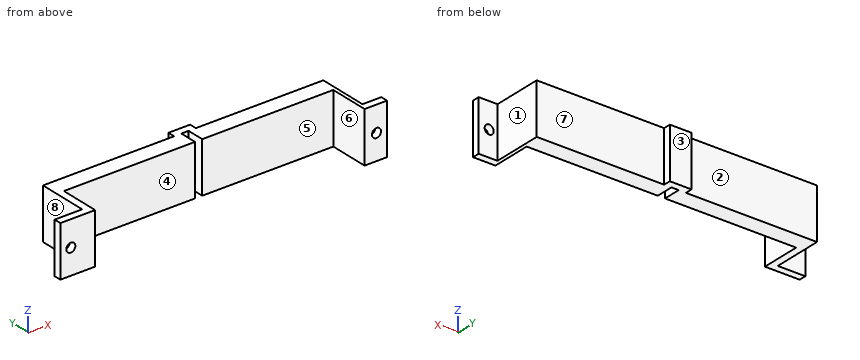
```python
from build123d import *

# Parameters (mm, degrees)
BOSS_EXTRUDE1_DEPTH = 17.78
SKETCH4_R           = 1.5875
CUT_EXTRUDE1_DEPTH  = 66.571859971


with BuildPart() as part:
    # Sketch3 → Boss-Extrude1 (new body)
    with BuildSketch(Plane.XY):
        Polygon((2.54, -2.54), (5.08, -2.54), (5.08, -8.636), (51.054, -8.636), (51.054, -22.606), (58.928, -22.606), (58.928, -20.066), (52.324, -20.066), (52.324, -2.54), (7.62, -2.54), (7.62, 0), (0, 0), (0, -2.54), (-45.974, -2.54), (-45.974, -20.066), (-55.626, -20.066), (-55.626, -22.606), (-43.434, -22.606), (-43.434, -8.636), (2.54, -8.636), align=None)
    extrude(amount=BOSS_EXTRUDE1_DEPTH)

    # Sketch4 → Cut-Extrude1 (cut, through all)
    with BuildSketch(Plane.XZ.offset(22.606)):
        with Locations(Location((-51.943, 8.839936473, 0), (0, 0, 270))):
            Circle(SKETCH4_R)
        with Locations(Location((55.245, 8.839936473, 0), (0, 0, 270))):
            Circle(SKETCH4_R)
    extrude(amount=-CUT_EXTRUDE1_DEPTH, mode=Mode.SUBTRACT)


solid = part.part
```
Geometry check sheet. Reference: the model listing, model coordinates, mm. Face numbers are marked on the shaded views. A direction names the side the tool comes from. Coordinates: 2 decimals unless noted, no trailing zeros. Order: outer loops, then holes, each group sorted by start corner. A loop starts at its lowest first (then second) coordinate and runs counter-clockwise, first axis right, second up.
Q1. Thickness scan on probe 1 along X at (y, z) = (-19.5, 6.5); probe 2 along X at (y, z) = (-8, 16); probe 3 along Y at (x, z) = (46, 3). Record the ranges inside material, lowest first.
Reply:
probe 1: x = -45.97 to -43.43, 51.05 to 52.32
probe 2: x = -45.97 to 2.54, 5.08 to 52.32
probe 3: y = -8.64 to -2.54
Q2. Sectioned sample at C-C on y = -15. Record the cut outline in (x, z), and give its area (3 significant figures).
Reply:
outline: (-45.97, 0) - (-43.43, 0) - (-43.43, 17.78) - (-45.97, 17.78) - close; (51.05, 0) - (52.32, 0) - (52.32, 17.78) - (51.05, 17.78) - close
area: 67.7 mm2
Q3. Sectioned sample at D-D on x = 3.5. Record the cut outline in (y, z), and give its area (3 significant figures).
Reply:
outline: (-2.54, 0) - (0, 0) - (0, 17.78) - (-2.54, 17.78) - close
area: 45.2 mm2
Q4. Sectioned sample at B-B on z = 6.25. Record the cut outline in (x, y), and give its area (3 significant figures).
Reply:
outline: (-55.63, -22.61) - (-43.43, -22.61) - (-43.43, -8.64) - (2.54, -8.64) - (2.54, -2.54) - (5.08, -2.54) - (5.08, -8.64) - (51.05, -8.64) - (51.05, -22.61) - (58.93, -22.61) - (58.93, -20.07) - (52.32, -20.07) - (52.32, -2.54) - (7.62, -2.54) - (7.62, 0) - (0, 0) - (0, -2.54) - (-45.97, -2.54) - (-45.97, -20.07) - (-55.63, -20.07) - close
area: 698 mm2
Q5. Depth check by flat-ended pin: pin 1 Ø5 at (x, z) = (-21, 13.5) entering from +Y; pin 2 Ø3 at (y, z) = (-7.5, 12.5) entering from -X; pin 3 Ø3 at (y, z) = (-6, 7) entering from +X. Enter the tip coordinate at first touch or a pass-through.
Reply:
pin 1: stops at y = -2.54
pin 2: stops at x = -45.97
pin 3: stops at x = 52.32
Q6. Sectioned sample at A-A on y = -6.75. Record the cut outline in (x, z).
Reply:
outline: (-45.97, 0) - (2.54, 0) - (2.54, 17.78) - (-45.97, 17.78) - close; (5.08, 0) - (52.32, 0) - (52.32, 17.78) - (5.08, 17.78) - close
Q7. Tool access check on the marked faces 1, 2, 3 and 4. Record the directions out of +Z, -Z, +X, -X, +Y, -Y that give a thin tool (end or side, any length) a straight path to the whole face; none if there is none.
Reply:
face 1: +Z, -Z, +X, +Y
face 2: +Z, -Z, -X, +Y
face 3: +Z, -Z, +X, -X, +Y
face 4: +Z, -Z, -Y
Q8. Draft check along X on the marked faces 5, 6, 7 and 8. Enter one of: released by +X, released by -X, zero draft, split by the parting line, or undercut.
Reply:
face 5: undercut
face 6: undercut
face 7: zero draft
face 8: released by -X
